from build123d import *

# Parameters (mm, degrees)
SALIENTE_EXTRUIR1_DEPTH = 46
REDONDEO1_R             = 1
CROQUIS2_R              = 2.85
CROQUIS2_R_2            = 5
CORTAR_EXTRUIR1_DEPTH   = 1
CORTAR_EXTRUIR2_DEPTH   = 88.669687299
CROQUIS6_R              = 5
CORTAR_EXTRUIR3_DEPTH   = 65.306026243
CROQUIS7_3_R            = 1.5
CROQUIS7_5_R            = 1.5
CROQUIS7_6_R            = 1.5
CORTAR_EXTRUIR4_DEPTH   = 64.501763056


with BuildPart() as part:
    # Croquis1 → Saliente-Extruir1 (new body)
    with BuildSketch(Plane.XY):
        with BuildLine():
            Line((-36.916417311, 3.674134953), (-36.916417311, -33.325865047))
            ThreePointArc((-36.916417311, -33.325865047), (-37.20931053, -34.032971828), (-37.916417311, -34.325865047))
            Line((-37.916417311, -34.325865047), (-65.916417311, -34.325865047))
            Line((-65.916417311, -34.325865047), (-65.916417311, -31.325865047))
            Line((-65.916417311, -31.325865047), (-40.916417311, -31.325865047))
            ThreePointArc((-40.916417311, -31.325865047), (-40.20931053, -31.032971828), (-39.916417311, -30.325865047))
            Line((-39.916417311, -30.325865047), (-39.916417311, 3.674134953))
            Line((-39.916417311, 3.674134953), (-36.916417311, 3.674134953))
        make_face()
    extrude(amount=SALIENTE_EXTRUIR1_DEPTH)

    # Redondeo1
    redondeo1_edges = [part.edges().sort_by_distance(p)[0] for p in [
        (-38.416417311, 3.674134953, 0),
        (-65.916417311, -32.825865047, 46),
        (-38.416417311, 3.674134953, 46),
        (-65.916417311, -32.825865047, 0),
    ]]
    fillet(redondeo1_edges, radius=REDONDEO1_R)

    # Croquis2 → Cortar-Extruir1 (cut)
    with BuildSketch(Plane.ZY.offset(36.916417311)):
        with Locations((6, -3.325865047)):
            Circle(CROQUIS2_R)
        with Locations((39, -3.325865047)):
            Circle(CROQUIS2_R)
        with Locations((6, -21.325865047)):
            Circle(CROQUIS2_R)
        with Locations((39, -21.325865047)):
            Circle(CROQUIS2_R)
        with Locations((15, -12.325865047)):
            Circle(CROQUIS2_R_2)
        with Locations((30, -12.325865047)):
            Circle(CROQUIS2_R_2)
    extrude(amount=CORTAR_EXTRUIR1_DEPTH, mode=Mode.SUBTRACT)

    # Croquis3 → Cortar-Extruir2 (cut, through all)
    with BuildSketch(Plane(origin=(0, -31.325865047, 0), x_dir=(1, 0, 0), z_dir=(0, 1, 0))):
        with BuildLine():
            Line((-62.916417311, -42), (-44.916417311, -42))
            ThreePointArc((-44.916417311, -42), (-42.916417311, -40), (-44.916417311, -38))
            Line((-44.916417311, -38), (-62.916417311, -38))
            ThreePointArc((-62.916417311, -38), (-64.916417311, -40), (-62.916417311, -42))
        make_face()
        with BuildLine():
            Line((-62.916417311, -9), (-44.916417311, -9))
            ThreePointArc((-44.916417311, -9), (-42.916417311, -7), (-44.916417311, -5))
            Line((-44.916417311, -5), (-62.916417311, -5))
            ThreePointArc((-62.916417311, -5), (-64.916417311, -7), (-62.916417311, -9))
        make_face()
    extrude(amount=-CORTAR_EXTRUIR2_DEPTH, mode=Mode.SUBTRACT)

    # Croquis6 → Cortar-Extruir3 (cut, through all)
    with BuildSketch(Plane(origin=(-36.916417311, 0, 0), x_dir=(0, 0, -1), z_dir=(1, 0, 0))):
        with Locations((-30, -12.325865047)):
            Circle(CROQUIS6_R)
        with Locations((-15, -12.325865047)):
            Circle(CROQUIS6_R)
    extrude(amount=-CORTAR_EXTRUIR3_DEPTH, mode=Mode.SUBTRACT)

    # Cortar-Recubrir1: read off the stored shape, not the designer's step
    # Cortar-Recubrir1: loft between two sections, ruled curve by curve
    cortar_recubrir1_from = [
        Edge.make_bspline([(-37.916417311, -6.071519474, 38.235878437), (-37.916417311, -7.599762601, 43.727187292), (-37.916417311, -2.108453745, 45.255430419), (-37.916417311, -0.580210619, 39.764121563), (-37.916417311, 0.948032507, 34.272812708), (-37.916417311, -4.543276348, 32.744569581), (-37.916417311, -6.071519474, 38.235878437)], [0, 0, 0, 0, 0.5, 0.5, 0.5, 1, 1, 1, 1], 3, [1, 0.333333333, 0.333333333, 1, 0.333333333, 0.333333333, 1]),
    ]
    cortar_recubrir1_to = [
        Edge.make_bspline([(-38.746417311, -4.801032854, 39.271808645), (-38.746417311, -4.257415563, 42.22214426), (-38.746417311, -1.307079948, 41.67852697), (-38.746417311, -1.850697239, 38.728191355), (-38.746417311, -2.39431453, 35.77785574), (-38.746417311, -5.344650145, 36.32147303), (-38.746417311, -4.801032854, 39.271808645)], [0, 0, 0, 0, 0.5, 0.5, 0.5, 1, 1, 1, 1], 3, [1, 0.333333333, 0.333333333, 1, 0.333333333, 0.333333333, 1]),
    ]
    cortar_recubrir1 = Solid(Shell([*[Face.make_surface_from_curves(cortar_recubrir1_from[k], cortar_recubrir1_to[k]) for k in range(1)], Face(Wire(cortar_recubrir1_from)), Face(Wire(cortar_recubrir1_to))]))
    add(cortar_recubrir1, mode=Mode.SUBTRACT)

    # Croquis7<3> → section 1 of cortar_recubrir2
    with BuildSketch(Plane(origin=(-38.746417311, 0, 0), x_dir=(0, 0, -1), z_dir=(1, 0, 0)), mode=Mode.PRIVATE) as cortar_recubrir2_s1:
        with Locations((-39, -21.325865047)):
            Circle(CROQUIS7_3_R)
    # loft up to a face of the part (cortar_recubrir2)
    loft([Face(Wire([part.edges().sort_by_distance((-37.916417311, -23.403425635, 37.049040748))[0]])), cortar_recubrir2_s1.sketch], mode=Mode.SUBTRACT)

    # Cortar-Recubrir3: read off the stored shape, not the designer's step
    # Cortar-Recubrir3: loft between two sections, ruled curve by curve
    cortar_recubrir3_from = [
        Edge.make_bspline([(-37.916417311, -24.050926068, 6.834591174), (-37.916417311, -22.38174372, 12.284713218), (-37.916417311, -16.931621677, 10.615530869), (-37.916417311, -18.600804025, 5.165408826), (-37.916417311, -20.269986373, -0.284713218), (-37.916417311, -25.720108417, 1.384469131), (-37.916417311, -24.050926068, 6.834591174)], [0, 0, 0, 0, 0.5, 0.5, 0.5, 1, 1, 1, 1], 3, [1, 0.333333333, 0.333333333, 1, 0.333333333, 0.333333333, 1]),
    ]
    cortar_recubrir3_to = [
        Edge.make_bspline([(-38.746417311, -22.643490638, 6.716842243), (-38.746417311, -21.209806151, 9.352093425), (-38.746417311, -18.574554969, 7.918408939), (-38.746417311, -20.008239456, 5.283157757), (-38.746417311, -21.441923942, 2.647906575), (-38.746417311, -24.077175124, 4.081591061), (-38.746417311, -22.643490638, 6.716842243)], [0, 0, 0, 0, 0.5, 0.5, 0.5, 1, 1, 1, 1], 3, [1, 0.333333333, 0.333333333, 1, 0.333333333, 0.333333333, 1]),
    ]
    cortar_recubrir3 = Solid(Shell([*[Face.make_surface_from_curves(cortar_recubrir3_from[k], cortar_recubrir3_to[k]) for k in range(1)], Face(Wire(cortar_recubrir3_from)), Face(Wire(cortar_recubrir3_to))]))
    add(cortar_recubrir3, mode=Mode.SUBTRACT)

    # Croquis7<5> → section 1 of cortar_recubrir4
    with BuildSketch(Plane(origin=(-38.746417311, 0, 0), x_dir=(0, 0, -1), z_dir=(1, 0, 0)), mode=Mode.PRIVATE) as cortar_recubrir4_s1:
        with Locations((-6, -3.325865047)):
            Circle(CROQUIS7_5_R)
    # loft up to a face of the part (cortar_recubrir4)
    loft([Face(Wire([part.edges().sort_by_distance((-37.916417311, -5.403425635, 4.049040748))[0]])), cortar_recubrir4_s1.sketch], mode=Mode.SUBTRACT)

    # Croquis7<6> → Cortar-Extruir4 (cut, through all)
    with BuildSketch(Plane(origin=(-38.746417311, 0, 0), x_dir=(0, 0, -1), z_dir=(1, 0, 0))):
        with Locations((-39, -3.325865047)):
            Circle(CROQUIS7_6_R)
        with Locations((-39, -21.325865047)):
            Circle(CROQUIS7_6_R)
        with Locations((-6, -21.325865047)):
            Circle(CROQUIS7_6_R)
        with Locations((-6, -3.325865047)):
            Circle(CROQUIS7_6_R)
    extrude(amount=-CORTAR_EXTRUIR4_DEPTH, mode=Mode.SUBTRACT)


solid = part.part
The listing builds one solid part. Answer for the finished solid, in the listing's coordinates (mm). A direction names the side the tool comes from. Give positions to 0.01 mm unless a question says otherwise; leave off trailing zeros. Order: outer loops, then holes, each group sorted by start corner. A loop starts at its lowest first (then second) coordinate and runs counter-clockwise, first axis right, second up. Notation, with made-up numbers: (56.5, 64.5) -> (103.5, 64.5) arc R12 cw to (103.5, 68.5) -> close; hole circle Ø7 at (25, 26). An arc over 180 degrees is marked (long way). Put each result on its own line as item: value.
Item 1: A cutting plane is placed at B-B on x = -59. Give the vertices of the cut face in (y, z), plus the area to 3 significant figures.
Established:
outline: (-34.33, 0) -> (-31.33, 0) -> (-31.33, 5) -> (-34.33, 5) -> close; (-34.33, 9) -> (-31.33, 9) -> (-31.33, 38) -> (-34.33, 38) -> close; (-34.33, 42) -> (-31.33, 42) -> (-31.33, 46) -> (-34.33, 46) -> close
area: 114 mm^2
Item 2: Straight lines are drawn through the part: line 1 (Y direction, x = -39, z = 6); line 2 (Z direction, x = -57.5, y = -32); line 3 (Y direction, x = -38.4, z = 30). For each, find the intervals that lie inside material, in ascending order.
Established:
line 1: y = -34.33 to -22.83, -19.83 to -4.83, -1.83 to 3.67
line 2: z = 0 to 5, 9 to 38, 42 to 46
line 3: y = -34.33 to -17.33, -7.33 to 3.67
Item 3: A cutting plane is placed at C-C on z = 29. Give the vertices of the cut face in (x, y).
Established:
outline: (-65.92, -34.33) -> (-37.92, -34.33) arc R1 ccw to (-36.92, -33.33) -> (-36.92, -17.22) -> (-39.92, -17.22) -> (-39.92, -30.33) arc R1 cw to (-40.92, -31.33) -> (-65.92, -31.33) -> close; (-39.92, -7.43) -> (-36.92, -7.43) -> (-36.92, 3.67) -> (-39.92, 3.67) -> close
Item 4: A cutting plane is placed at D-D on y = -27. Give the vertices of the cut face in (x, z), plus the area to 3 significant figures.
Established:
outline: (-39.92, 0) -> (-36.92, 0) -> (-36.92, 46) -> (-39.92, 46) -> close
area: 138 mm^2
Item 5: Given P1, Ø2, axis at y = -19, z = 30.5, coming from the -X side; P2, Ø8, axis at x = -45.5, z = 13, coming from the +Y side; P3, Ø3.5, axis at y = -21.33, z = 39, coming from the +X side; P4, Ø3, axis at x = -49, y = -29.5, coming from the +Z side, each flat-ended and moving along its own axis, determine where each tip first touches the part or whether it passes through.
Established:
P1: stops at x = -39.92
P2: stops at y = -31.33
P3: stops at x = -38.59
P4: passes through
Item 6: For a pull along Y with two mould halves and no side action, classify faces 1 (the face through (-38.4, 3.39, 0.3)), 2 (the face through (-39, -21, 0)), 3 (the face through (-37.41, -4.42, 8.63)) as released by +Y, released by -Y, zero draft, split by the parting line, or undercut.
Established:
face 1: released by +Y
face 2: zero draft
face 3: undercut
Item 7: For faces 4 (the face through (-39, -21, 46)), 5 (the face through (-54, -31.326, 23)), 6 (the face through (-54, -33, 42)), 7 (the face through (-37.41, -2.47, 41.72)), determine the directions among +Z, -Z, +X, -X, +Y, -Y from which every point of the face is accessible in a straight line to the end or side of a thin tool.
Established:
face 4: +Z, +X, -X, +Y, -Y
face 5: +Z, -Z, -X, +Y
face 6: +Y, -Y
face 7: +X
Item 8: A cutting plane is placed at A-A on z = 15. Give the vertices of the cut face in (x, y).
Established:
outline: (-65.92, -34.33) -> (-37.92, -34.33) arc R1 ccw to (-36.92, -33.33) -> (-36.92, -17.33) -> (-39.92, -17.33) -> (-39.92, -30.33) arc R1 cw to (-40.92, -31.33) -> (-65.92, -31.33) -> close; (-39.92, -7.33) -> (-36.92, -7.33) -> (-36.92, 3.67) -> (-39.92, 3.67) -> close
